Read the model definition and answer for the solid it produces. Units are mm, in the model's axes. A direction names the side the tool comes from. Coordinates: 2 decimals unless noted, no trailing zeros. Loops run counter-clockwise (first coordinate to the right, second up) from the corner with the lowest first, then second, coordinate; pieces in that order, holes last.
Q1. Which of the six approach directions +Z, -Z, +X, -X, +Y, -Y give full straight-line access (tool end or side, diameter ignored) to faces 1 (the face through (-3, 11, 45)), 2 (the face through (157, 10, 2))?
Q2. Section B-B (y = 15.25) is taken. Give the vertices of the cut face in (x, z), then the cut area to 3 significant figures.
Q3. Straight lines are drawn through the part: line 1 (Z direction, x = 0, y = 8.25); line 2 (X direction, y = 1.75, z = -4); line 3 (Z direction, x = 60, y = 14.5). For each, find the intervals that lie inside material, in ascending order.
Q4. A flat-ended cylindrical pin translates along its axis: P1, Ø16, axis at x = -1, z = 1, coming from the +Y side. Find the tip coordinate at first contact, or state that the pin passes through.
Q5. Section A-A (x = 150) is taken. Give the vertices of the cut face in (y, z), then the cut area to 4 significant figures.
Q6. The mould has two halves that part along Z. Classify faces 3 (the face through (-3, 0, -11)), 4 (the face through (1.46, 4.93, 6.59)), 5 (the face through (-3, 11, -45)): pulls with the +Z half, pulls with the -Z half, needs draft (parallel to the pull), parting line crosses it, or undercut.
Q7. Section C-C (z = 0) is taken. Count the separate pieces of the cut face and the enclosed holes in it, then the cut area to 4 significant figures.
from build123d import *

# Parameters (mm, degrees)
SKETCH_1_W                          = 370
SKETCH_1_H                          = 90
EXTRUDE_1_DEPTH                     = 23
HOLE_WIZARD_M4_1_D                  = 13.5
HOLE_WIZARD_M4_1_CBORE_D            = 20
HOLE_WIZARD_M4_1_CBORE_DEPTH        = 13
PATTERN_LINEAR_1_COUNT              = 2
PATTERN_LINEAR_1_PITCH              = 90
PATTERN_LINEAR_2_COPY_1_D           = 13.5
PATTERN_LINEAR_2_COPY_1_CBORE_D     = 20
PATTERN_LINEAR_2_COPY_1_CBORE_DEPTH = 13
PATTERN_LINEAR_2_COPY_2_D           = 13.5
PATTERN_LINEAR_2_COPY_2_CBORE_D     = 20
PATTERN_LINEAR_2_COPY_2_CBORE_DEPTH = 13
PATTERN_START                       = 10
PATTERN_LINEAR_3_OUTLINE_R          = 10
PATTERN_LINEAR_3_DEPTH              = 13
PATTERN_LINEAR_3_2_OUTLINE_R        = 6.75
PATTERN_LINEAR_3_2_DEPTH            = 10


# Read off the part's stored shape, not the designer's step: 阵列(线性)3
with BuildPart() as part:
    # 草图1 → 凸台-拉伸1 (new body)
    with BuildSketch(Plane(origin=(0, 0, 0), x_dir=(1, 0, 0), z_dir=(0, 1, 0))):
        Rectangle(SKETCH_1_W, SKETCH_1_H)
    extrude(amount=EXTRUDE_1_DEPTH)

    # M4 六角头螺栓的柱形沉头孔1 (through all)
    with Locations(Plane(origin=(0, 23, 0), x_dir=(1, 0, 0), z_dir=(0, 1, 0))):
        with Locations((-150, 0)):
            hole_wizard_m4_1 = CounterBoreHole(HOLE_WIZARD_M4_1_D / 2, HOLE_WIZARD_M4_1_CBORE_D / 2, HOLE_WIZARD_M4_1_CBORE_DEPTH)

    # 阵列(线性)1: M4 六角头螺栓的柱形沉头孔1 ×2
    with Locations(*[(i * PATTERN_LINEAR_1_PITCH, 0, 0) for i in range(1, PATTERN_LINEAR_1_COUNT)]):
        add(hole_wizard_m4_1, mode=Mode.SUBTRACT)

    # 阵列(线性)2 copy 1 (through all)
    with Locations(Plane(origin=(150, 23, 0), x_dir=(1, 0, 0), z_dir=(0, 1, 0))):
        with Locations((-150, 0)):
            CounterBoreHole(PATTERN_LINEAR_2_COPY_1_D / 2, PATTERN_LINEAR_2_COPY_1_CBORE_D / 2, PATTERN_LINEAR_2_COPY_1_CBORE_DEPTH)

    # 阵列(线性)2 copy 2 (through all)
    with Locations(Plane(origin=(210, 23, 0), x_dir=(1, 0, 0), z_dir=(0, 1, 0))):
        with Locations((-150, 0)):
            CounterBoreHole(PATTERN_LINEAR_2_COPY_2_D / 2, PATTERN_LINEAR_2_COPY_2_CBORE_D / 2, PATTERN_LINEAR_2_COPY_2_CBORE_DEPTH)

    # 阵列(线性)3 outline → 阵列(线性)3 (cut)
    with BuildSketch(Plane(origin=(0, 0, 0), x_dir=(1, 0, 0), z_dir=(0, 1, 0)).offset(PATTERN_START)):
        with Locations((150, 0)):
            Circle(PATTERN_LINEAR_3_OUTLINE_R)
    extrude(amount=PATTERN_LINEAR_3_DEPTH, mode=Mode.SUBTRACT)

    # Pattern Linear 3 2 outline → Pattern Linear 3 2 (cut)
    with BuildSketch(Plane(origin=(0, 0, 0), x_dir=(1, 0, 0), z_dir=(0, 1, 0))):
        with Locations((150, 0)):
            Circle(PATTERN_LINEAR_3_2_OUTLINE_R)
    extrude(amount=PATTERN_LINEAR_3_2_DEPTH, mode=Mode.SUBTRACT)


solid = part.part
Numbers:
1. face 1: +Z, +X, -X, +Y, -Y
1. face 2: +Y
2. outline: (-185, -45) - (185, -45) - (185, 45) - (-185, 45) - close; hole circle Ø20 at (-150, 0); hole circle Ø20 at (-60, 0); hole circle Ø20 at (0, 0); hole circle Ø20 at (60, 0); hole circle Ø20 at (150, 0)
2. area: 31,700 mm2
3. line 1: z = -45 to -6.75, 6.75 to 45
3. line 2: x = -185 to -155.44, -144.56 to -65.44, -54.56 to -5.44, 5.44 to 54.56, 65.44 to 144.56, 155.44 to 185
3. line 3: z = -45 to -10, 10 to 45
4. P1: stops at y = 10
5. outline: (0, -45) - (23, -45) - (23, -10) - (10, -10) - (10, -6.75) - (0, -6.75) - close; (0, 6.75) - (10, 6.75) - (10, 10) - (23, 10) - (23, 45) - (0, 45) - close
5. area: 1,675 mm2
6. face 3: needs draft
6. face 4: undercut
6. face 5: pulls with the -Z half
7. separate pieces: 6
7. enclosed holes: 0
7. area: 6,535 mm2
